Answer from the drawing. Dimensions are ordinates in mm from the lowest x, y and z of the part. A direction names the side the tool comes from. Round coordinates to 2 decimals unless told otherwise and drop trailing zeros. Order: outer loops, then holes, each group sorted by start corner. A loop starts at its lowest first (then second) coordinate and runs counter-clockwise, first axis right, second up. Notation, with made-up numbers: (74, 54) - (121, 54) arc R20 cw to (121, 80) - close; hole circle Ø2 at (-18, -10). An arc over 180 degrees is marked (long way). One line per question, with ' | ' between items. Start each with the question number.
1) The part is cut by section C-C, the plane x = 15.25. Give the vertices of the cut face in (y, z), plus the area to 3 significant figures.
2) The part is cut by section B-B, the plane z = 10. Give the vertices of the cut face in (x, y).
3) Flat-ended cylindrical pins translate along their axes: pin 1 (3 mm diameter, centred on x = 15, y = 8, fed in from +Z); pin 2 (14 mm diameter, centred on x = 19.5, y = 16, fed in from +Z); pin 3 (8 mm diameter, centred on x = 10.5, z = 8, fed in from -Y); pin 4 (6.5 mm diameter, centred on x = 15, y = 22, fed in from -Z). Find the tip coordinate at first contact, or state that the pin passes through.
4) For the marked faces 1 and 2, determine the directions among +Z, -Z, +X, -X, +Y, -Y from which every point of the face is accessible in a straight line to the end or side of a thin tool.
5) Straight lines are drawn through the part: line 1 (Y direction, x = 15, z = 1.2); line 2 (Y direction, x = 15, z = 0.7); line 3 (Z direction, x = 5.75, y = 2.5). For each, find the intervals that lie inside material, in ascending order. Write a range as from..to.
6) The part is cut by section D-D, the plane x = 7.5. Give the vertices of the cut face in (y, z).
7) The part is cut by section A-A, the plane y = 22. Give the vertices of the cut face in (x, z).
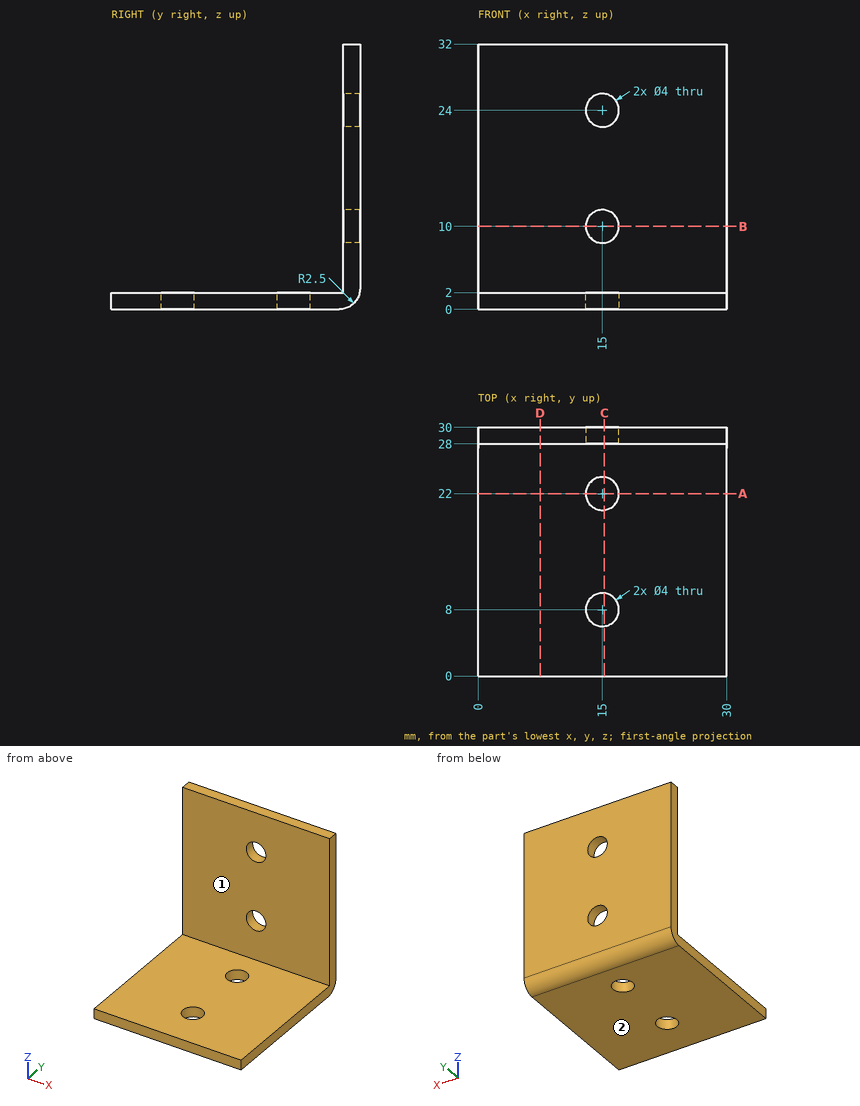
Values:
1) outline: (0, 0) - (6.02, 0) - (6.02, 2) - (0, 2) - close; (9.98, 0) - (20.02, 0) - (20.02, 2) - (9.98, 2) - close; (23.98, 0) - (27.5, 0) arc R2.5 ccw to (30, 2.5) - (30, 8.02) - (28, 8.02) - (28, 2) - (23.98, 2) - close; (28, 11.98) - (30, 11.98) - (30, 22.02) - (28, 22.02) - close; (28, 25.98) - (30, 25.98) - (30, 32) - (28, 32) - close | area: 86.9 mm^2
2) outline: (0, 28) - (13, 28) - (13, 30) - (0, 30) - close; (17, 28) - (30, 28) - (30, 30) - (17, 30) - close
3) pin 1: passes through | pin 2: stops at z = 2 | pin 3: stops at y = 28 | pin 4: stops at z = 0
4) face 1: +Z, +X, -X, -Y | face 2: -Z, +X, -X, +Y, -Y
5) line 1: y = 0..6, 10..20, 24..29.64 | line 2: y = 0..6, 10..20, 24..29.23 | line 3: z = 0..2
6) outline: (0, 0) - (27.5, 0) arc R2.5 ccw to (30, 2.5) - (30, 32) - (28, 32) - (28, 2) - (0, 2) - close
7) outline: (0, 0) - (13, 0) - (13, 2) - (0, 2) - close; (17, 0) - (30, 0) - (30, 2) - (17, 2) - close
